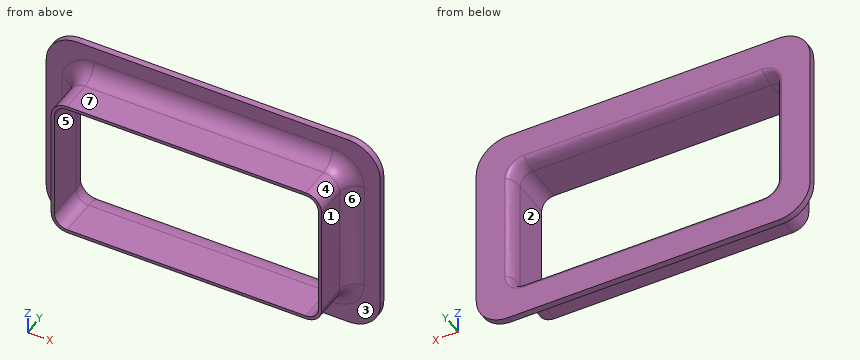
from build123d import *

# Parameters (mm, degrees)
BOSS_EXTRUDE1_DEPTH = 19.05
BOSS_EXTRUDE2_DEPTH = 2.54
FILLET1_R           = 6.35
FILLET3_SIZE        = 6.35
FILLET3_SIZE_2      = 2.54


with BuildPart() as part:
    # Sketch1 → Boss-Extrude1 (new body)
    with BuildSketch(Plane(origin=(0, 0, 0), x_dir=(1, 0, 0), z_dir=(0, 1, 0))):
        with BuildLine():
            Line((-47.625, 28.575), (47.625, 28.575))
            ThreePointArc((47.625, 28.575), (52.115128061, 26.715128061), (53.975, 22.225))
            Line((53.975, 22.225), (53.975, -22.225))
            ThreePointArc((53.975, -22.225), (52.115128061, -26.715128061), (47.625, -28.575))
            Line((47.625, -28.575), (-47.625, -28.575))
            ThreePointArc((-47.625, -28.575), (-52.115128061, -26.715128061), (-53.975, -22.225))
            Line((-53.975, -22.225), (-53.975, 22.225))
            ThreePointArc((-53.975, 22.225), (-52.115128061, 26.715128061), (-47.625, 28.575))
        make_face()
        with BuildLine():
            Line((-52.705, 22.225), (-52.705, -22.225))
            ThreePointArc((-52.705, -22.225), (-51.217102448, -25.817102448), (-47.625, -27.305))
            Line((-47.625, -27.305), (47.625, -27.305))
            ThreePointArc((47.625, -27.305), (51.217102448, -25.817102448), (52.705, -22.225))
            Line((52.705, -22.225), (52.705, 22.225))
            ThreePointArc((52.705, 22.225), (51.217102448, 25.817102448), (47.625, 27.305))
            Line((47.625, 27.305), (-47.625, 27.305))
            ThreePointArc((-47.625, 27.305), (-51.217102448, 25.817102448), (-52.705, 22.225))
        make_face(mode=Mode.SUBTRACT)
    extrude(amount=BOSS_EXTRUDE1_DEPTH)

    # Sketch2 → Boss-Extrude2 (add)
    with BuildSketch(Plane(origin=(0, 19.05, 0), x_dir=(1, 0, 0), z_dir=(0, 1, 0))):
        with BuildLine():
            Line((-53.975, -41.275), (53.975, -41.275))
            ThreePointArc((53.975, -41.275), (62.955256121, -37.555256121), (66.675, -28.575))
            Line((66.675, -28.575), (66.675, 28.575))
            ThreePointArc((66.675, 28.575), (62.955256121, 37.555256121), (53.975, 41.275))
            Line((53.975, 41.275), (-53.975, 41.275))
            ThreePointArc((-53.975, 41.275), (-62.955256121, 37.555256121), (-66.675, 28.575))
            Line((-66.675, 28.575), (-66.675, -28.575))
            ThreePointArc((-66.675, -28.575), (-62.955256121, -37.555256121), (-53.975, -41.275))
        make_face()
        with BuildLine():
            Line((52.705, -22.225), (52.705, 22.225))
            ThreePointArc((52.705, 22.225), (51.217102448, 25.817102448), (47.625, 27.305))
            Line((47.625, 27.305), (-47.625, 27.305))
            ThreePointArc((-47.625, 27.305), (-51.217102448, 25.817102448), (-52.705, 22.225))
            Line((-52.705, 22.225), (-52.705, -22.225))
            ThreePointArc((-52.705, -22.225), (-51.217102448, -25.817102448), (-47.625, -27.305))
            Line((-47.625, -27.305), (47.625, -27.305))
            ThreePointArc((47.625, -27.305), (51.217102448, -25.817102448), (52.705, -22.225))
        make_face(mode=Mode.SUBTRACT)
    extrude(amount=BOSS_EXTRUDE2_DEPTH)

    # Fillet1
    fillet1_edges = [part.edges().sort_by_distance(p)[0] for p in [
        (-52.115128061, 19.05, -26.715128061),
        (-53.975, 19.05, 0),
        (-52.115128061, 19.05, 26.715128061),
        (0, 19.05, 28.575),
        (52.115128061, 19.05, 26.715128061),
        (53.975, 19.05, 0),
        (52.115128061, 19.05, -26.715128061),
        (0, 19.05, -28.575),
    ]]
    fillet(fillet1_edges, radius=FILLET1_R)

    # Fillet3
    # an asymmetric fillet: 6.35, 2.54 mm, written as the material it takes off along each edge
    with BuildSketch(Plane(origin=(47.625, 21.59, -22.225), x_dir=(1, 0, 0), z_dir=(0, 0, 1))) as fillet3_piece_1:
        with BuildLine():
            Bezier((5.08, -FILLET3_SIZE), (5.08, 0), (5.08 + FILLET3_SIZE_2, 0), weights=[1, 0.707106781, 1])
            Line((5.08 + FILLET3_SIZE_2, 0), (5.08, 0))
            Line((5.08, 0), (5.08, -FILLET3_SIZE))
        make_face()
    revolve(axis=Axis((47.625, 21.59, -22.225), (0, 1, 0)), revolution_arc=90, mode=Mode.SUBTRACT)
    with BuildSketch(Plane(origin=(52.705, 21.59, 22.225), x_dir=(0, -1, 0), z_dir=(0, 0, -1)), Plane(origin=(-52.705, 21.59, -22.225), x_dir=(0, -1, 0), z_dir=(0, 0, 1))) as fillet3_piece_2:
        with BuildLine():
            Bezier((FILLET3_SIZE, 0), (0, 0), (0, -FILLET3_SIZE_2), weights=[1, 0.707106781, 1])
            Line((0, -FILLET3_SIZE_2), (0, 0))
            Line((0, 0), (FILLET3_SIZE, 0))
        make_face()
    extrude(amount=44.45, mode=Mode.SUBTRACT)
    with BuildSketch(Plane(origin=(47.625, 21.59, 22.225), x_dir=(0, 0, 1), z_dir=(-1, 0, 0))) as fillet3_piece_3:
        with BuildLine():
            Bezier((5.08, -FILLET3_SIZE), (5.08, 0), (5.08 + FILLET3_SIZE_2, 0), weights=[1, 0.707106781, 1])
            Line((5.08 + FILLET3_SIZE_2, 0), (5.08, 0))
            Line((5.08, 0), (5.08, -FILLET3_SIZE))
        make_face()
    revolve(axis=Axis((47.625, 21.59, 22.225), (0, 1, 0)), revolution_arc=90, mode=Mode.SUBTRACT)
    with BuildSketch(Plane(origin=(-47.625, 21.59, 27.305), x_dir=(0, -1, 0), z_dir=(1, 0, 0)), Plane(origin=(47.625, 21.59, -27.305), x_dir=(0, -1, 0), z_dir=(-1, 0, 0))) as fillet3_piece_4:
        with BuildLine():
            Bezier((FILLET3_SIZE, 0), (0, 0), (0, -FILLET3_SIZE_2), weights=[1, 0.707106781, 1])
            Line((0, -FILLET3_SIZE_2), (0, 0))
            Line((0, 0), (FILLET3_SIZE, 0))
        make_face()
    extrude(amount=95.25, mode=Mode.SUBTRACT)
    with BuildSketch(Plane(origin=(-47.625, 21.59, 22.225), x_dir=(-1, 0, 0), z_dir=(0, 0, -1))) as fillet3_piece_5:
        with BuildLine():
            Bezier((5.08, -FILLET3_SIZE), (5.08, 0), (5.08 + FILLET3_SIZE_2, 0), weights=[1, 0.707106781, 1])
            Line((5.08 + FILLET3_SIZE_2, 0), (5.08, 0))
            Line((5.08, 0), (5.08, -FILLET3_SIZE))
        make_face()
    revolve(axis=Axis((-47.625, 21.59, 22.225), (0, 1, 0)), revolution_arc=90, mode=Mode.SUBTRACT)
    with BuildSketch(Plane(origin=(-47.625, 21.59, -22.225), x_dir=(0, 0, -1), z_dir=(1, 0, 0))) as fillet3_piece_6:
        with BuildLine():
            Bezier((5.08, -FILLET3_SIZE), (5.08, 0), (5.08 + FILLET3_SIZE_2, 0), weights=[1, 0.707106781, 1])
            Line((5.08 + FILLET3_SIZE_2, 0), (5.08, 0))
            Line((5.08, 0), (5.08, -FILLET3_SIZE))
        make_face()
    revolve(axis=Axis((-47.625, 21.59, -22.225), (0, 1, 0)), revolution_arc=90, mode=Mode.SUBTRACT)


solid = part.part
Work out the finished part from the listing and answer in its coordinate system (mm). Face numbers are marked on the shaded views. A direction names the side the tool comes from. Give positions to 0.01 mm unless a question says otherwise; leave off trailing zeros. Order: outer loops, then holes, each group sorted by start corner. A loop starts at its lowest first (then second) coordinate and runs counter-clockwise, first axis right, second up. Notation, with made-up numbers: (-27, 82.5) -> (28, 82.5) arc R22 ccw to (28, 118.5) -> close; hole circle Ø10 at (-28, -24.5). An arc over 180 degrees is marked (long way). Answer as a JSON object with one key per item and string values. Group by question number.
1. Section A-A on y = 6.25 is taken. Determine the outline of the cut face in (x, z) (3 decimals), plus the area to 3 significant figures.
2. Flat-ended cylindrical pins translate along their axes: pin 1 Ø5 at (x, y) = (-38, 15.5) entering from +Z; pin 2 Ø1.5 at (y, z) = (5.5, 8) entering from +X (3 decimals); pin 3 Ø6.5 at (x, y) = (-4.5, 9.5) entering from +Z; pin 4 Ø25 at (x, z) = (26, 19.5) entering from -Y. Find the tip coordinate at first contact, or state that the pin passes through.
3. Consider line 1 along X through (y, z) = (4.5, -3) (3 decimals); line 2 along Z through (x, y) = (38, 5) (3 decimals); line 3 along Y through (x, z) = (-53, 38). Determine where each line is inside the solid, lowest interval first. Write a range as [from, to].
4. A tool of negligible diameter and unlimited length cuts with its end or side. For the marked faces 1, 2, 3 and 4, from which of +Z, -Z, +X, -X, +Y, -Y can it reach the whole face along a straight path? Write none if from no direction.
5. The mould has two halves that part along X. Classify the marked faces 5, 6 and 7: released by +X, released by -X, zero draft, split by the parting line, or undercut.
Result sheet:
{
 "1": {"outline": "(-53.975, -22.225) arc R6.35 ccw to (-47.625, -28.575) -> (47.625, -28.575) arc R6.35 ccw to (53.975, -22.225) -> (53.975, 22.225) arc R6.35 ccw to (47.625, 28.575) -> (-47.625, 28.575) arc R6.35 ccw to (-53.975, 22.225) -> close; hole (-52.705, -22.225) arc R5.08 ccw to (-47.625, -27.305) -> (47.625, -27.305) arc R5.08 ccw to (52.705, -22.225) -> (52.705, 22.225) arc R5.08 ccw to (47.625, 27.305) -> (-47.625, 27.305) arc R5.08 ccw to (-52.705, 22.225) -> close", "area": "400 mm^2"},
 "2": {"pin 1": "stops at z = 31.43", "pin 2": "stops at x = 53.975", "pin 3": "stops at z = 28.58", "pin 4": "stops at y = 0"},
 "3": {"line 1": "x = [-53.975, -52.705], [52.705, 53.975]", "line 2": "z = [-28.575, -27.305], [27.305, 28.575]", "line 3": "y = [19.05, 21.59]"},
 "4": {"face 1": "+Z, -Z, +X, -Y", "face 2": "+Y, -Y", "face 3": "-Y", "face 4": "+Z, +X, -Y"},
 "5": {"face 5": "undercut", "face 6": "released by +X", "face 7": "zero draft"}
}
